Part model, mm, in its own coordinate system. A direction names the side the tool comes from. Coordinates: 2 decimals unless noted, no trailing zeros. Order: outer loops, then holes, each group sorted by start corner. A loop starts at its lowest first (then second) coordinate and runs counter-clockwise, first axis right, second up. Notation, with made-up numbers: (53.5, 25.25) - (80.5, 25.25) arc R21 ccw to (80.5, 54.25) - close; hole circle Ø6 at (52, -23.5). An arc over 180 degrees is marked (long way). Use a Markdown table: item, result. Add a question column.
1) Two-plate mould, pull along Z, no slides. Class faces 5 (the face through (-1.5, 4.44, 0.07)), 6 (the face through (-12.5, 14, 0)), 7 (the face through (6.337, 14.437, 10.775)): +Z half, -Z half, draft (parallel to the pull), parting line (faces both ways), or undercut.
2) Saw through at A-A on z = -4.5. List the corners of the cut face in (x, y), then the cut area to 3 significant figures.
3) Saw through at C-C on x = -3.5. List the corners of the cut face in (y, z).
4) Saw through at B-B on y = 16. List the corners of the cut face in (x, z), then the cut area to 3 significant figures.
5) Drop flat-ended pins along their axis: P1, Ø6, axis at y = 12, z = 7.5, coming from the +X side; P2, Ø1, axis at x = 4.5, y = 10.5, coming from the +Z side; P3, Ø1.5, axis at x = 7, z = -11.5, coming from the +Y side (3 decimals); P4, Ø1.5, axis at x = 0, z = 0, coming from the -Y side. Give the stop position or say it passes through.
6) Saw through at D-D on z = 8.5. List the corners of the cut face in (x, y).
7) Wall check: L1, parallel to Z at x = 0, y = 5; L2, parallel to Y at x = 11.25, z = -7.25; L3, parallel to Z at x = 1.25, y = 7. Give the ranges that are in metal, low to high. Write a range as [from, to].
8) Tool access for faces 1 (the face through (5.5, 34, 0)), 2 (the face through (-5.5, 34, 0)), 3 (the face through (0, 34, -5.5)), 4 (the face through (-11, 19, 7)): list every direction of +Z, -Z, +X, -X, +Y, -Y with a clear straight run to the whole face (end or side of a thin tool).
Autodesk Inventor part; units mm, degrees
ref_plane "Work Plane1" through (0, 19, 0) normal (0.866, 0, 0.5) x (0, 1, 0)
ref_plane "XZ Plane" through (0, 0, 0) normal (0, 1, 0) x (-1, 0, 0)
ref_plane "XY Plane" through (0, 0, 0) normal (0, 0, 1) x (1, 0, 0)
sketch "Sketch2" plane through (0, 0, 0) normal (0, 1, 0) x (-1, 0, 0)
  circle A0 centre (0, 0) radius 5
  dimension "d0" = 10
extrude "Extrusion1" add sketch "Sketch2" along normal blind 10
sketch "Sketch3" plane through (0, 10, 0) normal (0, 1, 0) x (1, 0, 0)
  line L0 (0, -14.4338) -> (-12.5, -7.2169)
  line L1 (-12.5, -7.2169) -> (-12.5, 7.2169)
  line L2 (-12.5, 7.2169) -> (0, 14.4338)
  line L3 (0, 14.4338) -> (12.5, 7.2169)
  line L4 (12.5, 7.2169) -> (12.5, -7.2169)
  line L5 (12.5, -7.2169) -> (0, -14.4338)
  point P0 (0, 0)
  point P1 (0, 0)
  dimension "d14" = 25
extrude "Extrusion2" add sketch "Sketch3" along normal blind 9
sketch "Sketch4" plane through (0, 19, 0) normal (0, 1, 0) x (1, 0, 0)
  circle A0 centre (0, 0) radius 12.5
  line L0 (-12.5, -7.2169) -> (0, -14.4338)
extrude "Extrusion3" add sketch "Sketch4" along normal blind 10
sketch "Sketch5" plane through (0, 29, 0) normal (0, 1, 0) x (1, 0, 0)
  line L0 (5.5, -5.5) -> (-5.5, -5.5)
  line L1 (-5.5, -5.5) -> (-5.5, 5.5)
  line L2 (-5.5, 5.5) -> (5.5, 5.5)
  line L3 (5.5, 5.5) -> (5.5, -5.5)
  line L4 (5.5, -5.5) -> (-5.5, 5.5) construction
  line L5 (-5.5, -5.5) -> (5.5, 5.5) construction
  point P0 (0, 0)
  dimension "d7" = 11
  dimension "d8" = 11
extrude "Extrusion4" add sketch "Sketch5" along normal blind 10
thread "Thread1"
sketch "Sketch8" plane through (0, 0, 0) normal (0, -1, 0) x (1, 0, 0)
  circle A0 centre (0, 0) radius 1.5
  dimension "d24" = 3
extrude "Extrusion7" cut sketch "Sketch8" against normal blind 9
ref_plane "Work Plane1" through (0, 19, 0) normal (0.866, 0, 0.5) x (0, 1, 0)
equation "\"d8\" = d7"
properties part number "PressureSensor" material "Steel, Carbon"
Results are:
| question | item | result |
|---|---|---|
| 1 | face 5 | undercut |
| 1 | face 6 | draft |
| 1 | face 7 | +Z half |
| 2 | outline | (-12.5, 10) - (-2.18, 10) - (-2.18, 0) - (2.18, 0) - (2.18, 10) - (12.5, 10) - (12.5, 19) - (11.66, 19) - (11.66, 29) - (5.5, 29) - (5.5, 39) - (-5.5, 39) - (-5.5, 29) - (-11.66, 29) - (-11.66, 19) - (-12.5, 19) - close |
| 2 | area | 612 mm2 |
| 3 | outline | (0, -3.57) - (10, -3.57) - (10, -12.41) - (19, -12.41) - (19, -12) - (29, -12) - (29, -5.5) - (39, -5.5) - (39, 5.5) - (29, 5.5) - (29, 12) - (19, 12) - (19, 12.41) - (10, 12.41) - (10, 3.57) - (0, 3.57) - close |
| 4 | outline | (-12.5, -7.22) - (0, -14.43) - (12.5, -7.22) - (12.5, 7.22) - (0, 14.43) - (-12.5, 7.22) - close |
| 4 | area | 541 mm2 |
| 5 | P1 | x = 12.5 |
| 5 | P2 | z = 12.12 |
| 5 | P3 | through |
| 5 | P4 | y = 9 |
| 6 | outline | (-10.28, 10) - (10.28, 10) - (10.28, 19) - (9.17, 19) - (9.17, 29) - (-9.17, 29) - (-9.17, 19) - (-10.28, 19) - close |
| 7 | L1 | [-5, -1.5], [1.5, 5] |
| 7 | L2 | [10, 19] |
| 7 | L3 | [-4.84, -0.83], [0.83, 4.84] |
| 8 | face 1 | +Z, -Z, +X, +Y |
| 8 | face 2 | +Z, -Z, -X, +Y |
| 8 | face 3 | -Z, +X, -X, +Y |
| 8 | face 4 | +Z, -X, +Y |
